```python
from build123d import *

# Parameters (mm, degrees)
BOSS_EXTRUDE1_DEPTH            = 1
BOSS_EXTRUDE2_DEPTH            = 65
SKETCH4_W                      = 40
SKETCH4_H                      = 60
CUT_EXTRUDE1_DEPTH             = 1.5
SKETCH5_W                      = 35
SKETCH5_H                      = 55
CUT_EXTRUDE2_DEPTH             = 1.3
BOSS_EXTRUDE3_DEPTH            = 1
CUT_EXTRUDE3_REACH             = 75.478
CUT_EXTRUDE3_DIRECTION_2_REACH = 75.478
CUT_EXTRUDE4_DEPTH             = 0.6
CUT_EXTRUDE4_DIRECTION_2_REACH = 75.478
SKETCH8_R                      = 1
CUT_EXTRUDE5_DEPTH             = 1.3


with BuildPart() as part:
    # Sketch1 → Boss-Extrude1 (new body)
    with BuildSketch(Plane(origin=(0, 0, 0), x_dir=(1, 0, 0), z_dir=(0, 1, 0))):
        Polygon((23.261119363, -8.370540245), (15.148938036, 19.535999959), (-13.898560763, 20.444452223), (-23.738720982, -6.900633603), (-0.772775653, -24.709278334), align=None)
    extrude(amount=BOSS_EXTRUDE1_DEPTH)

    # Sketch2 → Boss-Extrude2 (add)
    with BuildSketch(Plane(origin=(0, 1, 0), x_dir=(1, 0, 0), z_dir=(0, 1, 0))):
        Polygon((-2.923895425, -23.04122038), (-0.772775653, -24.709278334), (-13.898560763, 20.444452223), (-14.820245584, 17.883157492), align=None)
        Polygon((-13.898560763, 20.444452223), (-0.772775653, -24.709278334), (0.270689735, -23.999909017), (-12.637422708, 20.405010489), align=None)
    extrude(amount=BOSS_EXTRUDE2_DEPTH)

    # Sketch4 → Cut-Extrude1 (cut)
    with BuildSketch(Plane(origin=(-8.872070504, 0, 2.579031444), x_dir=(0.2791364928440536, 0, 0.9602514349704049), z_dir=(-0.9602514349704049, 0, 0.2791364928440536))):
        with Locations((0, 33.5)):
            Rectangle(SKETCH4_W, SKETCH4_H)
    extrude(amount=-CUT_EXTRUDE1_DEPTH, mode=Mode.SUBTRACT)

    # Sketch5 → Cut-Extrude2 (cut)
    with BuildSketch(Plane(origin=(-7.431693352, 0, 2.160326705), x_dir=(0.2791364928440537, 0, 0.9602514349704049), z_dir=(-0.9602514349704049, 0, 0.2791364928440537))):
        with Locations((0, 33.5)):
            Rectangle(SKETCH5_W, SKETCH5_H)
    extrude(amount=-CUT_EXTRUDE2_DEPTH, mode=Mode.SUBTRACT)

    # Sketch7 → Boss-Extrude3 (add)
    with BuildSketch(Plane(origin=(0, 66, 0), x_dir=(1, 0, 0), z_dir=(0, 1, 0))):
        Polygon((-0.772775653, -24.709278334), (23.261119363, -8.370540245), (15.148938036, 19.535999959), (-13.898560763, 20.444452223), (-23.738720982, -6.900633603), align=None)
    extrude(amount=-BOSS_EXTRUDE3_DEPTH)

    # Cut-Extrude3: up to this face of the body (flat: up to its plane)
    cut_extrude3_end = Plane(part.part.faces().sort_by_distance((0, 66, 0))[0])
    # Sketch6 → Cut-Extrude3 (cut, up to the picked face)
    with BuildSketch(Plane(origin=(0, 1, 0), x_dir=(1, 0, 0), z_dir=(0, 1, 0)), mode=Mode.PRIVATE) as cut_extrude3_sk1:
        Polygon((-22.314397723, -6.486595587), (-5.107109693, -19.829764132), (-14.941634759, 14.001773661), align=None)
    cut_extrude3_tool1 = split(extrude(cut_extrude3_sk1.sketch, amount=CUT_EXTRUDE3_REACH, mode=Mode.PRIVATE), bisect_by=cut_extrude3_end, keep=Keep.BOTH, mode=Mode.PRIVATE)
    add(cut_extrude3_tool1.solids().sort_by(Axis((-14.121047, 1, 4.104862), (0, 1, 0)))[0], mode=Mode.SUBTRACT)

    # Cut-Extrude3 direction 2: up to this face of the body (flat: up to its plane)
    cut_extrude3_direction_2_end = Plane(part.part.faces().sort_by_distance((0, 0, 0))[0])
    # Sketch6 → Cut-Extrude3 direction 2 (cut, up to the picked face)
    with BuildSketch(Plane(origin=(0, 1, 0), x_dir=(1, 0, 0), z_dir=(0, 1, 0)), mode=Mode.PRIVATE) as cut_extrude3_direction_2_sk1:
        Polygon((-22.314397723, -6.486595587), (-5.107109693, -19.829764132), (-14.941634759, 14.001773661), align=None)
    cut_extrude3_direction_2_tool1 = split(extrude(cut_extrude3_direction_2_sk1.sketch, amount=-CUT_EXTRUDE3_DIRECTION_2_REACH, mode=Mode.PRIVATE), bisect_by=cut_extrude3_direction_2_end, keep=Keep.BOTH, mode=Mode.PRIVATE)
    add(cut_extrude3_direction_2_tool1.solids().sort_by(Axis((-14.121047, 1, 4.104862), (0, -1, 0)))[0], mode=Mode.SUBTRACT)

    # Sketch3 → Cut-Extrude4 (cut)
    with BuildSketch(Plane(origin=(0, 1, 0), x_dir=(1, 0, 0), z_dir=(0, 1, 0))):
        with BuildLine():
            Line((10.293293236, 12.233810418), (15.358065736, -5.038944994))
            ThreePointArc((15.358065736, -5.038944994), (8.914963643, -16.828195836), (-2.874287199, -10.385093743))
            Line((-2.874287199, -10.385093743), (-7.939059699, 6.887661669))
            ThreePointArc((-7.939059699, 6.887661669), (-1.495957606, 18.676912511), (10.293293236, 12.233810418))
        make_face()
    extrude(amount=-CUT_EXTRUDE4_DEPTH, mode=Mode.SUBTRACT)

    # Cut-Extrude4 direction 2: up to this face of the body (flat: up to its plane)
    cut_extrude4_direction_2_end = Plane(part.part.faces().sort_by_distance((2.593442955, 66, -0.753890642))[0])
    # Sketch3 → Cut-Extrude4 direction 2 (cut, up to the picked face)
    with BuildSketch(Plane(origin=(0, 1, 0), x_dir=(1, 0, 0), z_dir=(0, 1, 0)), mode=Mode.PRIVATE) as cut_extrude4_direction_2_sk1:
        with BuildLine():
            Line((10.293293236, 12.233810418), (15.358065736, -5.038944994))
            ThreePointArc((15.358065736, -5.038944994), (8.914963643, -16.828195836), (-2.874287199, -10.385093743))
            Line((-2.874287199, -10.385093743), (-7.939059699, 6.887661669))
            ThreePointArc((-7.939059699, 6.887661669), (-1.495957606, 18.676912511), (10.293293236, 12.233810418))
        make_face()
    cut_extrude4_direction_2_tool1 = split(extrude(cut_extrude4_direction_2_sk1.sketch, amount=CUT_EXTRUDE4_DIRECTION_2_REACH, mode=Mode.PRIVATE), bisect_by=cut_extrude4_direction_2_end, keep=Keep.BOTH, mode=Mode.PRIVATE)
    add(cut_extrude4_direction_2_tool1.solids().sort_by(Axis((3.709503, 1, -0.924358), (0, 1, 0)))[0], mode=Mode.SUBTRACT)

    # Sketch8 → Cut-Extrude5 (cut)
    with BuildSketch(Plane(origin=(-7.431693352, 0, 2.160326705), x_dir=(0.2791364928440537, 0, 0.9602514349704049), z_dir=(-0.9602514349704049, 0, 0.2791364928440537))):
        with Locations((-18.75, 4.75)):
            Circle(SKETCH8_R)
        with Locations((18.75, 4.75)):
            Circle(SKETCH8_R)
        with Locations((-18.75, 62.25)):
            Circle(SKETCH8_R)
        with Locations((18.75, 62.25)):
            Circle(SKETCH8_R)
    extrude(amount=-CUT_EXTRUDE5_DEPTH, mode=Mode.SUBTRACT)


solid = part.part
```
Geometry: final body of the model. Coordinates: model frame, mm. A direction names the side the tool comes from. Round coordinates to 2 decimals unless told otherwise and drop trailing zeros. Order: outer loops, then holes, each group sorted by start corner. A loop starts at its lowest first (then second) coordinate and runs counter-clockwise, first axis right, second up. Notation, with made-up numbers: (-8.5, -27) - (45.5, -27) arc R18 ccw to (45.5, -21) - close; hole circle Ø4 at (26, 61). An arc over 180 degrees is marked (long way). Use CSV: the item, a comma, the result in double quotes. Start each with the question number.
Q1. Section query B-B (x = 8). Return loops of the section in (y, z), and give its area (3 significant figures).
Q2. First-contact query: pin 1 (12 mm diameter, centred on x = -8, z = 3, fed in from -Y); pin 2 (10 mm diameter, centred on x = 1, y = 36.5, fed in from -Z); pin 3 (11 mm diameter, centred on x = 3, z = -1.5, fed in from +Y). Flat tips, straight axial feed; report the tip coordinate or a pass-through.
Q3. Section query A-A (y = 29). Return loops of the section in (x, z), and give its area (3 significant figures).
Q4. Mould query, pull axis X, two halves, no side actions, for faces 1 (the face through (19.26, 0.49, -5.39)), 2 (the face through (-9.5, 65, 4)), 3 (the face through (-2.579, 33.08, 21.578)), 4 (the face through (9.11, 0.7, 16.77)). Classes: +X half, -X half, draft (parallel to the pull), parting line (faces both ways), or undercut.
Q5. Section query C-C (z = 0). State how many separate pieces and enclosed holes the cut face has, and give its area (3 significant figures).
Q6. Access query for faces 5 (the face through (13.2, 65, -3.2)), 6 (the face through (9.11, 65.49, 16.77)), 7 (the face through (-9.956, 0.507, 3.151)). Directions: +Z, -Z, +X, -X, +Y, -Y. A direction counts if a zero-diameter tool reaches every point of the face in a straight line with its end or side. Return the directions, or none.
Q7. Material intervals for line 1 along Y through (x, z) = (18.5, 9.5); line 2 along Y through (x, z) = (-9.5, 0); line 3 along Y through (x, z) = (-2, -7), sorted ascending. Write a range as from..to.
Result set:
1,outline,"(0, -19.76) - (1, -19.76) - (1, -16.17) - (0.4, -16.17) - (0.4, 17.05) - (1, 17.05) - (1, 18.75) - (0, 18.75) - close; (65, -19.76) - (66, -19.76) - (66, -16.17) - (65, -16.17) - close; (65, 17.05) - (66, 17.05) - (66, 18.75) - (65, 18.75) - close"
1,area,"23.9 mm2"
2,pin 1,"stops at y = 0"
2,pin 2,"stops at z = 18.6"
2,pin 3,"stops at y = 0.4"
3,outline,"(-14.82, -17.88) - (-13.9, -20.44) - (-12.64, -20.41) - (-11.07, -15.01) - (-12.32, -14.64) - (-13.01, -17.04) - (-14.45, -16.63) - close; (-3.29, 21.78) - (-1.85, 21.37) - (-2.55, 18.96) - (-1.3, 18.6) - (0.27, 24) - (-0.77, 24.71) - (-2.92, 23.04) - close"
3,area,"22.2 mm2"
4,face 1,"+X half"
4,face 2,"draft"
4,face 3,"-X half"
4,face 4,"undercut"
5,separate pieces,"5"
5,enclosed holes,"0"
5,area,"52.7 mm2"
6,face 5,"-Z, +X"
6,face 6,"+Y"
6,face 7,"+Y, -Y"
7,line 1,"y = 0..1, 65..66"
7,line 2,"y = 0..3.5, 63.5..66"
7,line 3,"y = 0..0.4"
